Geometry: final body of the model. Coordinates: model frame, mm. A direction names the side the tool comes from. Give positions to 0.01 mm unless a question says otherwise; leave off trailing zeros. Loops run counter-clockwise (first coordinate to the right, second up) from the corner with the lowest first, then second, coordinate; pieces in that order, holes last. Notation, with made-up numbers: M -21.75,32 L 20.25,32 A29 ccw 20.25,71 Z; hole C 40,32.25 d5. An arc over 180 degrees is marked long. Put each result on its own line as item: value.
```python
from build123d import *
from OCP.BRepFilletAPI import BRepFilletAPI_MakeChamfer

# Parameters (mm, degrees)
BOSS_EXTRUDE1_DEPTH        = 10
BOSS_EXTRUDE2_DEPTH        = 12
CUT_EXTRUDE3_DEPTH         = 6
CUT_EXTRUDE3_DEPTH_BACK    = 14
SKETCH7_R                  = 1.95
SKETCH8_R                  = 1.95
CUT_EXTRUDE4_DEPTH         = 4
SKETCH9_R                  = 1.5
CUT_EXTRUDE5_DEPTH         = 4
LPATTERN1_COUNT            = 2
LPATTERN1_PITCH            = 75
CHAMFER2_SIZE              = 5.5
CHAMFER2_SIZE2             = 9
CHAMFER3_SIZE              = 7
CHAMFER3_SIZE2             = 2
LPATTERN2_COUNT            = 3
LPATTERN2_PITCH            = 75
SZKIC1_W                   = 22.668374216
SZKIC1_H                   = 5
WYTNIJ_WYCI_GNI_CIE1_DEPTH = 30.5


with BuildPart() as part:
    # Sketch1 → Boss-Extrude1 (new body)
    with BuildSketch(Plane(origin=(0, 0, 0), x_dir=(1, 0, 0), z_dir=(0, 1, 0))):
        with BuildLine():
            Line((0, -8.075), (0, -31.5))
            Line((0, -31.5), (22, -31.5))
            Line((22, -31.5), (22, 181.5))
            Line((22, 181.5), (0, 181.5))
            Line((0, 181.5), (0, 158.075))
            ThreePointArc((0, 158.075), (8.075, 150), (0, 141.925))
            Line((0, 141.925), (0, 83.075))
            ThreePointArc((0, 83.075), (8.075, 75), (0, 66.925))
            Line((0, 66.925), (0, 8.075))
            ThreePointArc((0, 8.075), (8.075, 0), (0, -8.075))
        make_face()
    extrude(amount=-BOSS_EXTRUDE1_DEPTH)

    # Sketch3 → Boss-Extrude2 (add)
    with BuildSketch(Plane.XZ.offset(10)):
        with BuildLine():
            Line((0, -181.5), (0, -158.075))
            ThreePointArc((0, -158.075), (8.075, -150), (0, -141.925))
            Line((0, -141.925), (0, -83.075))
            ThreePointArc((0, -83.075), (8.075, -75), (0, -66.925))
            Line((0, -66.925), (0, -8.075))
            ThreePointArc((0, -8.075), (8.075, 0), (0, 8.075))
            Line((0, 8.075), (0, 31.5))
            Line((0, 31.5), (5, 31.5))
            Line((5, 31.5), (5, 12.081209583))
            ThreePointArc((5, 12.081209583), (13.075, 0), (5, -12.081209583))
            Line((5, -12.081209583), (5, -62.918790417))
            ThreePointArc((5, -62.918790417), (13.075, -75), (5, -87.081209583))
            Line((5, -87.081209583), (5, -137.918790417))
            ThreePointArc((5, -137.918790417), (13.075, -150), (5, -162.081209583))
            Line((5, -162.081209583), (5, -181.5))
            Line((5, -181.5), (0, -181.5))
        make_face()
    extrude(amount=BOSS_EXTRUDE2_DEPTH)

    # Sketch7 → Cut-Extrude3 (cut, two sides: drawn at the far end of the back side and taken through both)
    with BuildSketch(Plane.ZY.offset(-CUT_EXTRUDE3_DEPTH_BACK)):
        with Locations((-170.5, -4)):
            Circle(SKETCH7_R)
        with Locations((-170.5, -18)):
            Circle(SKETCH7_R)
        with Locations(Location((-129.5, -4, 0), (0, 0, 180))):
            Circle(SKETCH7_R)
        with Locations((-129.5, -18)):
            Circle(SKETCH7_R)
        with Locations((-95.5, -4)):
            Circle(SKETCH7_R)
        with Locations(Location((-54.5, -4, 0), (0, 0, 180))):
            Circle(SKETCH7_R)
        with Locations((-54.5, -18)):
            Circle(SKETCH7_R)
        with Locations((-95.5, -18)):
            Circle(SKETCH7_R)
        with Locations((-20.5, -4)):
            Circle(SKETCH7_R)
        with Locations(Location((20.5, -4, 0), (0, 0, 180))):
            Circle(SKETCH7_R)
        with Locations((20.5, -18)):
            Circle(SKETCH7_R)
        with Locations((-20.5, -18)):
            Circle(SKETCH7_R)
    extrude(amount=CUT_EXTRUDE3_DEPTH + CUT_EXTRUDE3_DEPTH_BACK, mode=Mode.SUBTRACT)

    # Sketch8 → Cut-Extrude4 (cut)
    with BuildSketch(Plane.ZY):
        with Locations((-112.5, -18.5)):
            Circle(SKETCH8_R)
    cut_extrude4 = extrude(amount=-CUT_EXTRUDE4_DEPTH, mode=Mode.SUBTRACT)

    # Sketch9 → Cut-Extrude5 (cut)
    with BuildSketch(Plane.ZY.offset(-4)):
        with Locations((-112.5, -18.5)):
            Circle(SKETCH9_R)
    cut_extrude5 = extrude(amount=-CUT_EXTRUDE5_DEPTH, mode=Mode.SUBTRACT)

    # LPattern1: Cut-Extrude4, Cut-Extrude5 ×2
    with Locations(*[(0, 0, i * LPATTERN1_PITCH) for i in range(1, LPATTERN1_COUNT)]):
        add(cut_extrude4, mode=Mode.SUBTRACT)
        add(cut_extrude5, mode=Mode.SUBTRACT)

    # Chamfer2
    chamfer2_edges = [part.edges().sort_by_distance(p)[0] for p in [
        (22, -10, -75),
    ]]
    chamfer2_side = [part.faces().sort_by_distance(p)[0] for p in [
        (14.183508734, -10, -75),
    ]]
    chamfer(chamfer2_edges, length=CHAMFER2_SIZE, length2=CHAMFER2_SIZE2, reference=chamfer2_side[0])

    # Chamfer3: one chamfer whose edges measure the first distance from different faces: ONE call of the kernel's chamfer builder (chamfer() names one face for all edges)
    chamfer3_edges_1 = [part.edges().sort_by_distance(p)[0] for p in [
        (8.075, -22, 0),
    ]]
    chamfer3_side_1 = [part.faces().sort_by_distance(p)[0] for p in [
        (8.075, -11, 0),
    ]]
    chamfer3_edges_2 = [part.edges().sort_by_distance(p)[0] for p in [
        (8.075, -22, -75),
    ]]
    chamfer3_side_2 = [part.faces().sort_by_distance(p)[0] for p in [
        (8.075, -11, -75),
    ]]
    chamfer3_edges_3 = [part.edges().sort_by_distance(p)[0] for p in [
        (8.075, -22, -150),
    ]]
    chamfer3_side_3 = [part.faces().sort_by_distance(p)[0] for p in [
        (8.075, -11, -150),
    ]]
    chamfer3 = BRepFilletAPI_MakeChamfer(part.part.solid().wrapped)
    for e in chamfer3_edges_1:
        chamfer3.Add(CHAMFER3_SIZE, CHAMFER3_SIZE2, e.wrapped, chamfer3_side_1[0].wrapped)  # the first distance lies on this face
    for e in chamfer3_edges_2:
        chamfer3.Add(CHAMFER3_SIZE, CHAMFER3_SIZE2, e.wrapped, chamfer3_side_2[0].wrapped)  # the first distance lies on this face
    for e in chamfer3_edges_3:
        chamfer3.Add(CHAMFER3_SIZE, CHAMFER3_SIZE2, e.wrapped, chamfer3_side_3[0].wrapped)  # the first distance lies on this face
    add(Compound.cast(chamfer3.Shape()), mode=Mode.REPLACE)

    # Sketch10 → Cut-Revolve1 (revolve, cut)
    with BuildSketch(Plane.ZY):
        with BuildLine():
            Line((-159.575, 1.581763394), (-159.575, -1.5))
            ThreePointArc((-159.575, -1.5), (-157.014339828, -2.560660172), (-158.075, 0))
            Line((-158.075, 0), (-159.575, 1.581763394))
        make_face()
    cut_revolve1 = revolve(axis=Axis((0, 2.197765982, -150), (0, -1, 0)), mode=Mode.SUBTRACT)

    # LPattern2: Cut-Revolve1 ×3
    with Locations(*[(0, 0, i * LPATTERN2_PITCH) for i in range(1, LPATTERN2_COUNT)]):
        add(cut_revolve1, mode=Mode.SUBTRACT)

    # Szkic1 → Wytnij-wyciągnięcie1 (cut)
    with BuildSketch(Plane(origin=(0, 0, 0), x_dir=(1, 0, 0), z_dir=(0, 1, 0))):
        with Locations((11.334187108, -29)):
            Rectangle(SZKIC1_W, SZKIC1_H)
    extrude(amount=-WYTNIJ_WYCI_GNI_CIE1_DEPTH, mode=Mode.SUBTRACT)


solid = part.part
```
Item 1: Section B-B on z = -102.5. Output: boundary loops of the cut face in (x, y), then the cut area to 3 significant figures.
Output values:
outline: M 0,-22 L 5,-22 L 5,-10 L 16.5,-10 L 22,-1 L 22,0 L 0,0 Z
area: 255 mm²
Item 2: Set-up query: faces 5 (the flat face through (14, -4, -21)), 6 (the flat face through (8, -6, 26.5)), 7 (the cylindrical face through (9.573, -0.761, -0.211)). Return all of +Z, -Z, +X, -X, +Y, -Y with unobstructed straight access to the full face (end or side cutting, diameter ignored); none if empty.
Output values:
face 5: -X
face 6: +Z, +X, -X, +Y, -Y
face 7: -X, +Y
Item 3: Line query: probe 1 along Y at (x, z) = (1.3, -129.5); probe 2 along Z at (x, y) = (5.25, -14.5); probe 3 along Y at (x, z) = (14.25, -150). Output: solid intervals per line, ascending. Write a range as [from, to].
Output values:
probe 1: [-22, -19.95], [-16.05, -5.95], [-2.05, 0]
probe 2: [-161.97, -156.14], [-143.86, -138.03], [-86.97, -81.14], [-68.86, -63.03], [-11.97, -6.14], [6.14, 11.97]
probe 3: [-10, 0]
Item 4: Pin query (flat end, axial travel): pin 1 Ø6 at (y, z) = (-14, -173) entering from +X; pin 2 Ø1.9 at (y, z) = (-18, -38) entering from -X; pin 3 Ø5 at (y, z) = (-4, -20.5) entering from +X. Return the tip coordinate at first contact, or that it passes through.
Output values:
pin 1: x = 5
pin 2: x = 4
pin 3: x = 21.69
Item 5: Section A-A on z = -20.5. Output: boundary loops of the cut face in (x, y), then the cut area to 3 significant figures.
Output values:
outline: M 0,-22 L 5,-22 L 5,-19.95 L 0,-19.95 Z; M 0,-16.05 L 5,-16.05 L 5,-10 L 16.5,-10 L 22,-1 L 22,0 L 0,0 L 0,-2.05 L 14,-2.05 L 14,-5.95 L 0,-5.95 Z
area: 181 mm²
Item 6: Mould query, pull axis Y, two halves, no side actions, for faces 1 (the cylindrical face through (7.098, -4.086, 22.448)), 2 (the flat face through (19.289, -5.437, -76.044)), 3 (the flat face through (11, 0, -79)), 4 (the flat face through (5, -16, -37)). Classes: pulls with the +Y half, pulls with the -Y half, needs draft (parallel to the pull), parting line crosses it, or undercut.
Output values:
face 1: undercut
face 2: pulls with the -Y half
face 3: pulls with the +Y half
face 4: needs draft
